Can you work these out from the drawing? Everything is in mm from the part's minimum corner. A direction names the side the tool comes from. Coordinates: 2 decimals unless noted, no trailing zeros. Order: outer loops, then holes, each group sorted by start corner. A loop starts at its lowest first (then second) coordinate and runs counter-clockwise, first axis right, second up. Notation, with made-up numbers: (-21, 63) - (-15, 63) arc R20 cw to (-15, 92) - close; hole circle Ø5 at (-26.75, 82). An arc over 180 degrees is marked (long way). Answer as CSV lines item,"result". Start each with the question number.
Item 1: We'd pull the mould along X, two halves only. Please class the marked faces 4, 5, 6 and 7: pulls with the +X half, pulls with the -X half, needs draft (parallel to the pull), parting line crosses it, or undercut.
Item 2: Imagine slicing it at C-C on x = 5. List the corners of the cut face in (y, z) for me (1 decimal).
Item 3: I'm going to push flat-ended pins straight in: pin 1 (1.5 mm diameter, centred on y = 14, z = 1.5, fed in from -X); pin 2 (1.5 mm diameter, centred on y = 9.5, z = 6.5, fed in from +X) (1 decimal); pin 3 (2 mm diameter, centred on x = 9, y = 11.5, fed in from +Z); pin 4 (5.5 mm diameter, centred on x = 8.999, y = 3, fed in from +Z). Where does each tip first touch, or does it pass through?
Item 4: Imagine slicing it at A-A on z = 0.5. List the corners of the cut face in (x, y) for me.
Item 5: I need wall thicknesses on line 1 (Z direction, x = 10.5, y = 7); line 2 (Z direction, x = 3, y = 13); line 3 (Y direction, x = 7, z = 7). Which ranges of each line are inside material? Lowest first, please.
Item 6: Imagine slicing it at B-B on y = 3.25. List the corners of the cut face in (x, z) for me.
Item 7: On a 3-axis mill with a long thin cutter (end or side, diameter ignored), from which of +Z, -Z, +X, -X, +Y, -Y can I reach the whole of each face in a straight line? I mean the marked faces 1, 2 and 3. Say none if no direction works.
Item 8: Imagine slicing it at D-D on y = 10.25. List the corners of the cut face in (x, z) for me (1 decimal).
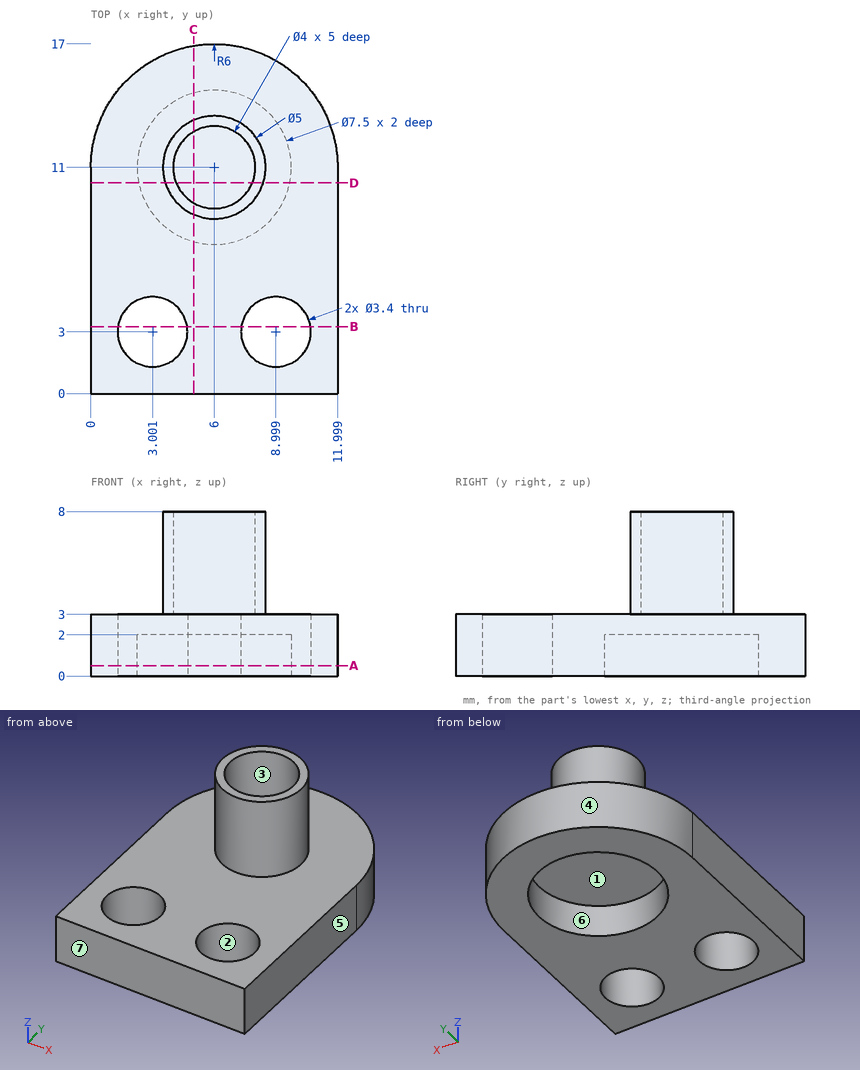
Responses:
1,face 4,"parting line crosses it"
1,face 5,"pulls with the +X half"
1,face 6,"undercut"
1,face 7,"needs draft"
2,outline,"(0, 0) - (7.4, 0) - (7.4, 2) - (14.6, 2) - (14.6, 0) - (16.9, 0) - (16.9, 3) - (13.3, 3) - (13.3, 8) - (12.7, 8) - (12.7, 3) - (9.3, 3) - (9.3, 8) - (8.7, 8) - (8.7, 3) - (0, 3) - close"
3,pin 1,"stops at x = 0.44"
3,pin 2,"stops at x = 8.4"
3,pin 3,"stops at z = 8"
3,pin 4,"stops at z = 3"
4,outline,"(0, 0) - (12, 0) - (12, 11) arc R6 ccw to (0, 11) - close; hole circle Ø3.4 at (3, 3); hole circle Ø7.5 at (6, 11); hole circle Ø3.4 at (9, 3)"
5,line 1,"z = 0 to 3"
5,line 2,"z = 2 to 3"
5,line 3,"y = 8.71 to 9.27, 12.73 to 13.29"
6,outline,"(0, 0) - (1.32, 0) - (1.32, 3) - (0, 3) - close; (4.68, 0) - (7.32, 0) - (7.32, 3) - (4.68, 3) - close; (10.68, 0) - (12, 0) - (12, 3) - (10.68, 3) - close"
7,face 1,"-Z"
7,face 2,"+Z, -Z"
7,face 3,"+Z"
8,outline,"(0, 0) - (2.3, 0) - (2.3, 2) - (9.7, 2) - (9.7, 0) - (12, 0) - (12, 3) - (8.4, 3) - (8.4, 8) - (7.9, 8) - (7.9, 3) - (4.1, 3) - (4.1, 8) - (3.6, 8) - (3.6, 3) - (0, 3) - close"
